The listing builds one solid part. Answer for the finished solid, in the listing's coordinates (mm). A direction names the side the tool comes from. Give positions to 0.01 mm unless a question says otherwise; leave off trailing zeros. Order: outer loops, then holes, each group sorted by start corner. A loop starts at its lowest first (then second) coordinate and runs counter-clockwise, first axis right, second up. Notation, with made-up numbers: (-5, 65.5) - (40, 65.5) arc R24 cw to (40, 87.5) - close; hole circle Ø5 at (52, 34). An arc over 180 degrees is marked (long way). Use a Markdown table: item, result. Add a question column.
1) Find section D-D, the plane y = -43. Determine the outline of the cut face in (x, z).
2) Flat-ended cylindrical pins translate along their axes: pin 1 (5 mm diameter, centred on y = -131, z = 3, fed in from +X); pin 2 (3 mm diameter, centred on x = -1.5, y = -139.5, fed in from -Z) (3 decimals); pin 3 (5 mm diameter, centred on x = 9, y = -149, fed in from -Z). Find the tip coordinate at first contact, or state that the pin passes through.
3) Find section C-C, the plane y = -178. Determine the outline of the cut face in (x, z) (3 decimals), plus the area to 3 significant figures.
4) Straight lines are drawn through the part: line 1 (Y direction, x = 6, z = 19.5); line 2 (Z direction, x = 1, y = -104); line 3 (Z direction, x = 10, y = -41.5). For each, find the intervals that lie inside material, in ascending order.
5) Find section B-B, the plane x = 0. Determine the outline of the cut face in (y, z) (3 decimals), plus the area to 3 significant figures.
6) For faces 1 (the face through (-4.16, -122.96, -18.74)), 2 (the face through (0, 0, 0)), determine the directions among +Z, -Z, +X, -X, +Y, -Y from which every point of the face is accessible in a straight line to the end or side of a thin tool.
7) Find section A-A, the plane z = 0. Determine the outline of the cut face in (x, y) (3 decimals), plus the area to 3 significant figures.
from build123d import *

# Parameters (mm, degrees)
F0_R     = 25.14462
F1_DEPTH = 50
F2_R     = 19.195006
F3_DEPTH = 150
F4_R     = 2
F5_R     = 5


with BuildPart() as f1:
    # F0 (on Front) → F1 (new body)
    with BuildSketch(Plane.XZ):
        Circle(F0_R)
    extrude(amount=F1_DEPTH)

    # F2 (on face) → F3 (join)
    with BuildSketch(Plane.XZ.offset(50)):
        Circle(F2_R)
    extrude(amount=F3_DEPTH)

    # F4
    f4_edges = [f1.edges().sort_by_distance(p)[0] for p in [
        (-19.195006, -200, 0),
        (-25.14462, 0, 0),
    ]]
    fillet(f4_edges, radius=F4_R)

    # F5
    f5_edges = [f1.edges().sort_by_distance(p)[0] for p in [
        (-25.14462, -50, 0),
    ]]
    fillet(f5_edges, radius=F5_R)


solid = f1.part
The answers:
| question | item | result |
|---|---|---|
| 1 | outline | circle Ø50.29 at (0, 0) |
| 2 | pin 1 | x = 19.19 |
| 2 | pin 2 | z = -19.195 |
| 2 | pin 3 | z = -18.06 |
| 3 | outline | circle Ø38.39 at (0, 0) |
| 3 | area | 1,160 mm2 |
| 4 | line 1 | -49.99 to 0 |
| 4 | line 2 | -19.17 to 19.17 |
| 4 | line 3 | -23.07 to 23.07 |
| 5 | outline | (-200, -17.195) arc R2 ccw to (-198, -19.195) - (-50, -19.195) - (-50, -20.145) arc R5 ccw to (-45, -25.145) - (-2, -25.145) arc R2 ccw to (0, -23.145) - (0, 23.145) arc R2 ccw to (-2, 25.145) - (-45, 25.145) arc R5 ccw to (-50, 20.145) - (-50, 19.195) - (-198, 19.195) arc R2 ccw to (-200, 17.195) - close |
| 5 | area | 8,260 mm2 |
| 6 | face 1 | -Y |
| 6 | face 2 | +Z, -Z, +X, -X, +Y |
| 7 | outline | (-25.145, -45) arc R5 ccw to (-20.145, -50) - (-19.195, -50) - (-19.195, -198) arc R2 ccw to (-17.195, -200) - (17.195, -200) arc R2 ccw to (19.195, -198) - (19.195, -50) - (20.145, -50) arc R5 ccw to (25.145, -45) - (25.145, -2) arc R2 ccw to (23.145, 0) - (-23.145, 0) arc R2 ccw to (-25.145, -2) - close |
| 7 | area | 8,260 mm2 |
